Verification items for the finished model (mm, model axes). Round coordinates to 2 decimals unless told otherwise and drop trailing zeros. Loops run counter-clockwise (first coordinate to the right, second up) from the corner with the lowest first, then second, coordinate; pieces in that order, holes last. Notation, with made-up numbers: (40.5, 56) -> (80.5, 56) arc R30 ccw to (80.5, 87) -> close; hole circle Ø10 at (30, 38.5). An arc over 180 degrees is marked (long way). Use a Markdown table: item, result. Add a question column.
```python
from build123d import *

# Parameters (mm, degrees)
F0_R     = 5.8945377359
F0_W     = 20.9622308612
F0_H     = 20.3956845216
F1_DEPTH = 30


with BuildPart() as f1:
    # F0 (on Front) → F1 (new body)
    with BuildSketch(Plane.XZ):
        Polygon((-36.967176944, -26.2027885765), (-36.6839058697, -46.3152006269), (-16.0049460828, -46.3152006269), (-16.0049460828, -26.2027885765), align=None)
        with Locations((-26.769336313, -36.4006310701)):
            Circle(F0_R, mode=Mode.SUBTRACT)
        with Locations((-26.4860615134, -16.0049463157)):
            Rectangle(F0_W, F0_H)
    extrude(amount=F1_DEPTH)


solid = f1.part
```
1) Release check for a two-part mould opening along Z. For faces 1 (the face through (-26, -15, -46.315)), 2 (the face through (-31.447, -14.79, -39.987)), 3 (the face through (-36.967, -15, -16)), 4 (the face through (-27, -15, -5.807)) record: released by +Z, released by -Z, zero draft, split by the parting line, or undercut.
2) Thickness scan on line 1 (Z direction, x = -23.25, y = -26.75); line 2 (Z direction, x = -29, y = -6.5); line 3 (X direction, y = -4.5, z = -36). Record the ranges inside material, lowest first.
3) Sectioned sample at B-B on x = -31.5. Enter the section's corners in (y, z), then the cut area to 3 significant figures.
4) Sectioned sample at A-A on z = -34.5. Enter the section's corners in (x, y).
5) Sectioned sample at C-C on y = -7. Enter the section's corners in (x, z), then the cut area to 3 significant figures.
Geometry results:
| question | item | result |
|---|---|---|
| 1 | face 1 | released by -Z |
| 1 | face 2 | undercut |
| 1 | face 3 | zero draft |
| 1 | face 4 | released by +Z |
| 2 | line 1 | -46.32 to -41.13, -31.67 to -5.81 |
| 2 | line 2 | -46.32 to -41.86, -30.94 to -5.81 |
| 2 | line 3 | -36.83 to -32.65, -20.89 to -16 |
| 3 | outline | (-30, -46.32) -> (0, -46.32) -> (0, -39.92) -> (-30, -39.92) -> close; (-30, -32.88) -> (0, -32.88) -> (0, -5.81) -> (-30, -5.81) -> close |
| 3 | area | 1,000 mm^2 |
| 4 | outline | (-36.85, -30) -> (-32.35, -30) -> (-32.35, 0) -> (-36.85, 0) -> close; (-21.19, -30) -> (-16, -30) -> (-16, 0) -> (-21.19, 0) -> close |
| 5 | outline | (-36.97, -26.2) -> (-36.68, -46.32) -> (-16, -46.32) -> (-16, -5.81) -> (-36.97, -5.81) -> close; hole circle Ø11.79 at (-26.77, -36.4) |
| 5 | area | 737 mm^2 |
